Can you work these out from the model? Positions are in its coordinate system, mm. Round coordinates to 2 decimals unless told otherwise and drop trailing zeros. Order: outer loops, then holes, each group sorted by start corner. A loop starts at its lowest first (then second) coordinate and runs counter-clockwise, first axis right, second up. Notation, with made-up numbers: (29, 41.5) -> (81, 41.5) arc R31 cw to (81, 78.5) -> close; hole circle Ø4 at (81.25, 10.25). An arc over 180 degrees is marked (long way). Use a Markdown table: item, result. Add a question column.
Q1. I need wall thicknesses on line 1 along Y through (x, z) = (-0.05, -0.5); line 2 along Z through (x, y) = (-0.05, -0.5); line 3 along Z through (x, y) = (-0.85, -1). Which ranges of each line are inside material? Lowest first, please. Write a range as [from, to].
Q2. If we section it at A-A on z = 2.6: List the corners of the cut face in (x, y) for me.
Q3. I'm going to push flat-ended pins straight in: pin 1 Ø0.7 at (x, z) = (0, 0.5) entering from -Y; pin 2 Ø1 at (x, y) = (-0.5, 3) entering from +Z. Where does each tip first touch, or does it pass through?
Q4. If we section it at C-C on x = -0.6: List the corners of the cut face in (y, z) for me, plus the area to 3 significant figures.
Q5. If we section it at D-D on x = 0.9: List the corners of the cut face in (y, z) for me, plus the area to 3 significant figures.
Q6. If we section it at B-B on y = -1.75: List the corners of the cut face in (x, z) for me, plus the area to 3 significant figures.
```python
from build123d import *

# Parameters (mm, degrees)
SKETCH2_R                = 1.1
BOSS_EXTRUDE1_DEPTH      = 3
BOSS_EXTRUDE1_DEPTH_BACK = 3
SWEEP1_PROFILE_R         = 0.2


with BuildPart() as part:
    # Sketch2 → Boss-Extrude1 (new body, two sides)
    with BuildSketch(Plane(origin=(0, 0, 0), x_dir=(1, 0, 0), z_dir=(0, 1, 0))) as boss_extrude1_sk:
        Circle(SKETCH2_R)
    extrude(amount=BOSS_EXTRUDE1_DEPTH)
    extrude(boss_extrude1_sk.sketch, amount=-BOSS_EXTRUDE1_DEPTH_BACK)

    # Sweep1: sweep along a path in Sketch3
    with BuildLine(Plane(origin=(0, 0, 0), x_dir=(0, 0, -1), z_dir=(1, 0, 0))) as sweep1_path:
        Line((0, 3), (0, 3.98))
        ThreePointArc((0, 3.98), (-0.322182541, 4.757817459), (-1.1, 5.08))
        Line((-1.1, 5.08), (-3.1, 5.08))
    # Sweep1 profile (on start of the path) → Sweep1 (sweep)
    with BuildSketch(Plane.ZX.offset(3)):
        Circle(SWEEP1_PROFILE_R)
    sweep1 = sweep(path=sweep1_path.line)

    # Mirror1: Sweep1 across plane
    add(sweep1.mirror(Plane.ZX))


solid = part.part
```
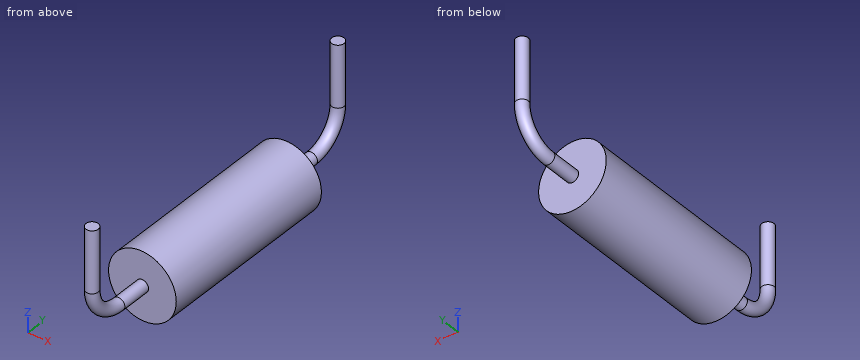
Answer below:
| question | item | result |
|---|---|---|
| 1 | line 1 | [-3, 3] |
| 1 | line 2 | [-1.1, 1.1] |
| 1 | line 3 | [-0.7, 0.7] |
| 2 | outline | circle Ø0.4 at (0, -5.08); circle Ø0.4 at (0, 5.08) |
| 3 | pin 1 | y = -5.26 |
| 3 | pin 2 | z = 1.1 |
| 4 | outline | (-3, -0.92) -> (3, -0.92) -> (3, 0.92) -> (-3, 0.92) -> close |
| 4 | area | 11.1 mm² |
| 5 | outline | (-3, -0.63) -> (3, -0.63) -> (3, 0.63) -> (-3, 0.63) -> close |
| 5 | area | 7.59 mm² |
| 6 | outline | circle Ø2.2 at (0, 0) |
| 6 | area | 3.80 mm² |
